Geometry check sheet. Reference: drawing and pictorial views, mm from the part's lowest x, y, z. A direction names the side the tool comes from. Round coordinates to 2 decimals unless told otherwise and drop trailing zeros. Order: outer loops, then holes, each group sorted by start corner. A loop starts at its lowest first (then second) coordinate and runs counter-clockwise, first axis right, second up. Notation, with made-up numbers: M -33.75,48.5 L 5.25,48.5 A18 ccw 5.25,71.5 Z; hole C 13,87.5 d2. An arc over 180 degrees is marked long. Answer as a JSON object with one key per item and string values. Group by question number.
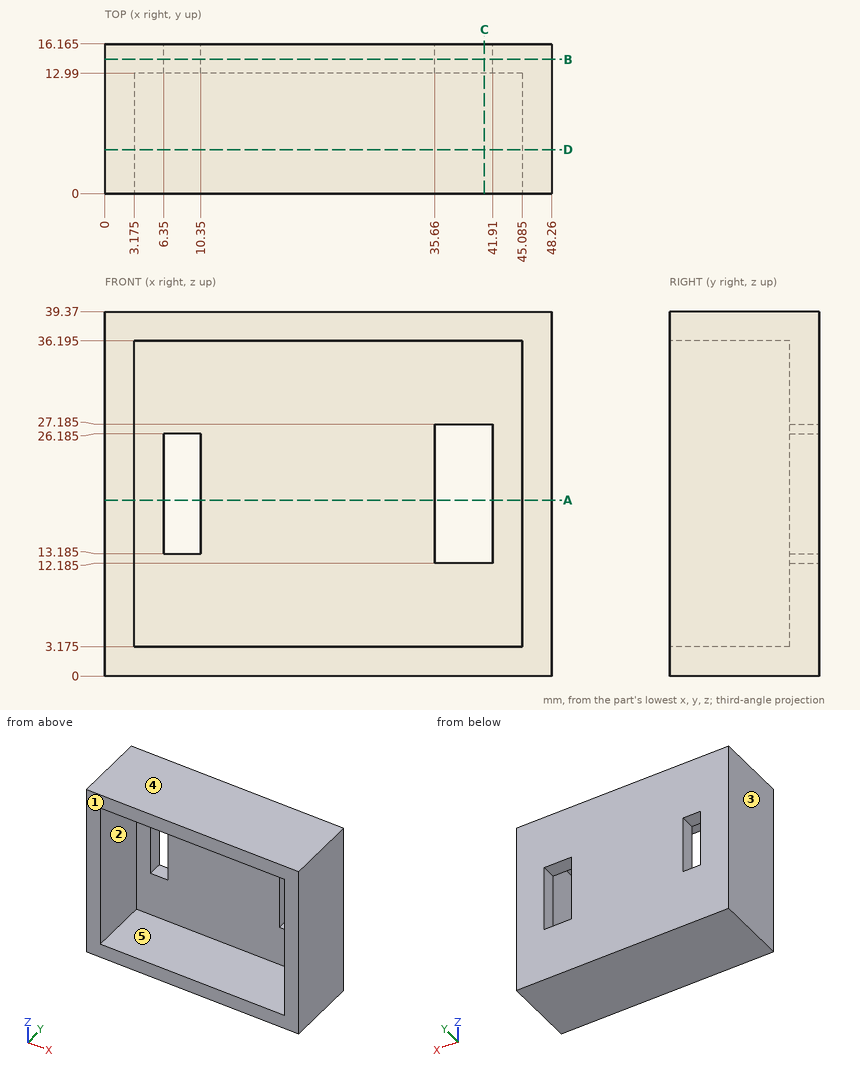
Q1. Release check for a two-part mould opening along Z. For the marked faces 3, 4 and 5 record: released by +Z, released by -Z, zero draft, split by the parting line, or undercut.
Q2. Thickness scan on line 1 (X direction, y = 9, z = 23.5) (3 decimals); line 2 (Z direction, x = 41.5, y = 4.5) (3 decimals); line 3 (X direction, y = 13.5, z = 27). Record the ranges inside material, lowest first. Write a range as from..to.
Q3. Cross-section at B-B, the plane y = 14.5. Record the cut outline in (x, z) (3 decimals).
Q4. Gauge pin test, flat end, axial feed: pin 1 Ø5 at (x, z) = (33.5, 29) entering from -Y. Record the tip position at first contact, or that the pin passes through.
Q5. Cross-section at C-C, the plane x = 41. Record the cut outline in (y, z) (1 decimal).
Q6. Tool access check on the marked faces 1 and 2. Record the directions out of +Z, -Z, +X, -X, +Y, -Y that give a thin tool (end or side, any length) a straight path to the whole face; none if there is none.
Q7. Cross-section at A-A, the plane z = 19. Give the number of separate pieces and of enclosed holes in the cut face, then the cut area to 3 significant figures.
Q8. Cross-section at D-D, the plane y = 4.75. Record the cut outline in (x, z) (3 decimals).
Conclusion:
{
 "1": {"face 3": "zero draft", "face 4": "released by +Z", "face 5": "undercut"},
 "2": {"line 1": "0..3.175, 45.085..48.26", "line 2": "0..3.175, 36.195..39.37", "line 3": "0..35.66, 41.91..48.26"},
 "3": {"outline": "M 0,0 L 48.26,0 L 48.26,39.37 L 0,39.37 Z; hole M 6.35,13.185 L 10.35,13.185 L 10.35,26.185 L 6.35,26.185 Z; hole M 35.66,12.185 L 41.91,12.185 L 41.91,27.185 L 35.66,27.185 Z"},
 "4": {"pin 1": "y = 12.99"},
 "5": {"outline": "M 0,0 L 16.2,0 L 16.2,12.2 L 13,12.2 L 13,3.2 L 0,3.2 Z; M 0,36.2 L 13,36.2 L 13,27.2 L 16.2,27.2 L 16.2,39.4 L 0,39.4 Z"},
 "6": {"face 1": "+Z, -Z, +X, -X, -Y", "face 2": "-Y"},
 "7": {"separate pieces": "3", "enclosed holes": "0", "area": "203 mm2"},
 "8": {"outline": "M 0,0 L 48.26,0 L 48.26,39.37 L 0,39.37 Z; hole M 3.175,3.175 L 45.085,3.175 L 45.085,36.195 L 3.175,36.195 Z"}
}
